```python
from build123d import *

# Parameters (mm, degrees)
SKETCH1_W           = 100
SKETCH1_H           = 200.1518
BOSS_EXTRUDE1_DEPTH = 6.35
SKETCH2_W           = 6.35
SKETCH2_H           = 50.8
SKETCH2_H_2         = 49.2759
CUT_EXTRUDE1_DEPTH  = 6.35
SKETCH3_W           = 61.9
SKETCH3_H           = 174.7518
CUT_EXTRUDE2_DEPTH  = 6.35
FILLET1_R           = 12.7


with BuildPart() as part:
    # Sketch1 → Boss-Extrude1 (new body)
    with BuildSketch(Plane.XY):
        with Locations((0, -50.0759)):
            Rectangle(SKETCH1_W, SKETCH1_H)
    extrude(amount=BOSS_EXTRUDE1_DEPTH)

    # Sketch2 → Cut-Extrude1 (cut)
    with BuildSketch(Plane.XY.offset(6.35)):
        with Locations((-46.825, -24.6759)):
            Rectangle(SKETCH2_W, SKETCH2_H)
        with Locations((-46.825, -75.4759)):
            Rectangle(SKETCH2_W, SKETCH2_H)
        with Locations((46.825, 25.36205)):
            Rectangle(SKETCH2_W, SKETCH2_H_2)
        with Locations((46.825, -125.51385)):
            Rectangle(SKETCH2_W, SKETCH2_H_2)
    extrude(amount=-CUT_EXTRUDE1_DEPTH, mode=Mode.SUBTRACT)

    # Sketch3 → Cut-Extrude2 (cut)
    with BuildSketch(Plane.XY.offset(6.35)):
        with Locations((0, -50.0759)):
            Rectangle(SKETCH3_W, SKETCH3_H)
    extrude(amount=-CUT_EXTRUDE2_DEPTH, mode=Mode.SUBTRACT)

    # Fillet1
    fillet1_edges = [part.edges().sort_by_distance(p)[0] for p in [
        (-30.95, -137.4518, 3.175),
        (-30.95, 37.3, 3.175),
        (30.95, 37.3, 3.175),
        (30.95, -137.4518, 3.175),
    ]]
    fillet(fillet1_edges, radius=FILLET1_R)


solid = part.part
```
Work out the finished part from the listing and answer in its coordinate system (mm). A direction names the side the tool comes from. Coordinates: 2 decimals unless noted, no trailing zeros. Loops run counter-clockwise (first coordinate to the right, second up) from the corner with the lowest first, then second, coordinate; pieces in that order, holes last. Notation, with made-up numbers: M -14,-32.5 L 11,-32.5 A15 ccw 11,-21.5 Z; hole C 86.5,52 d11. An arc over 180 degrees is marked long. Use CSV: the item, a comma, the result in double quotes. Start each with the question number.
(1) Given pin 1 Ø3 at (y, z) = (32, 3) entering from +X; pin 2 Ø3 at (y, z) = (-24.5, 4.5) entering from -X; pin 3 Ø3 at (x, z) = (47, 2.5) entering from -Y, each flat-ended and moving along its own axis, determine where each tip first touches the part or whether it passes through.
(2) For a pull along X with two mould halves and no side action, classify faces 5 (the face through (-50, 25, 3)), 6 (the face through (-47, -100.876, 3)), 7 (the face through (27.33, 33.48, 3.13)) as +X half, -X half, draft (parallel to the pull), parting line (faces both ways), or undercut.
(3) Find section B-B, the plane x = 6. Give the vertices of the cut face in (y, z).
(4) Find section C-C, the plane z = 4.5. Give the vertices of the cut face in (x, y).
(5) Find section A-A, the plane y = -2.5. Give the vertices of the cut face in (x, z), then the cut area to 3 significant figures.
(6) For faces 1 (the face through (43.65, 25, 3)), 2 (the face through (43.65, -126, 3)), 3 (the face through (-47, 0.724, 3)), 4 (the face through (0, -137.452, 3)), determine the directions among +Z, -Z, +X, -X, +Y, -Y from which every point of the face is accessible in a straight line to the end or side of a thin tool.
(7) Consider line 1 (X direction, y = -84, z = 1.25); line 2 (X direction, y = 19, z = 4.5); line 3 (Y direction, x = -44.5, z = 6.25). Determine where each line is inside the solid, lowest interval first.
Recorded:
1,pin 1,"stops at x = 43.65"
1,pin 2,"stops at x = -43.65"
1,pin 3,"stops at y = -100.88"
2,face 5,"-X half"
2,face 6,"draft"
2,face 7,"undercut"
3,outline,"M -150.15,0 L -137.45,0 L -137.45,6.35 L -150.15,6.35 Z; M 37.3,0 L 50,0 L 50,6.35 L 37.3,6.35 Z"
4,outline,"M -50,-150.15 L 43.65,-150.15 L 43.65,-100.88 L 50,-100.88 L 50,0.72 L 43.65,0.72 L 43.65,50 L -50,50 L -50,0.72 L -43.65,0.72 L -43.65,-100.88 L -50,-100.88 Z; hole M -30.95,-124.75 A12.7 ccw -18.25,-137.45 L 18.25,-137.45 A12.7 ccw 30.95,-124.75 L 30.95,24.6 A12.7 ccw 18.25,37.3 L -18.25,37.3 A12.7 ccw -30.95,24.6 Z"
5,outline,"M -43.65,0 L -30.95,0 L -30.95,6.35 L -43.65,6.35 Z; M 30.95,0 L 50,0 L 50,6.35 L 30.95,6.35 Z"
5,area,"202 mm^2"
6,face 1,"+Z, -Z, +X, +Y"
6,face 2,"+Z, -Z, +X, -Y"
6,face 3,"+Z, -Z, -X"
6,face 4,"+Z, -Z"
7,line 1,"x = -43.65 to -30.95, 30.95 to 50"
7,line 2,"x = -50 to -30.95, 30.95 to 43.65"
7,line 3,"y = -150.15 to -100.88, 0.72 to 50"
